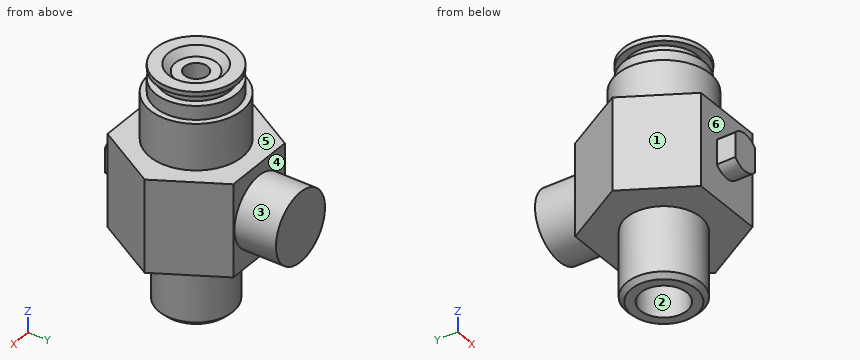
```python
from build123d import *

# Parameters (mm, degrees)
BOSS_EXTRUDE1_DEPTH = 20
SKETCH2_R           = 10
BOSS_EXTRUDE2_DEPTH = 10
SKETCH3_R           = 8.75
BOSS_EXTRUDE3_DEPTH = 6
SKETCH5_R           = 2.5
CUT_EXTRUDE1_DEPTH  = 18.5
SKETCH6_W           = 1.5
SKETCH6_H           = 2
SKETCH7_R           = 4
BOSS_EXTRUDE4_DEPTH = 4
CUT_EXTRUDE2_DEPTH  = 4
SKETCH9_R           = 7.5
BOSS_EXTRUDE5_DEPTH = 9
SKETCH10_R          = 8
SKETCH10_R_2        = 5
BOSS_EXTRUDE6_DEPTH = 15
CHAMFER1_SIZE       = 1


with BuildPart() as part:
    # Sketch1 → Boss-Extrude1 (new body)
    with BuildSketch(Plane.XY):
        Polygon((-7.875, 13.63990011), (7.875, 13.63990011), (15.75, 0), (7.875, -13.63990011), (-7.875, -13.63990011), (-15.75, 0), align=None)
    extrude(amount=BOSS_EXTRUDE1_DEPTH)

    # Sketch2 → Boss-Extrude2 (add)
    with BuildSketch(Plane.XY.offset(20)):
        Circle(SKETCH2_R)
    extrude(amount=BOSS_EXTRUDE2_DEPTH)

    # Sketch3 → Boss-Extrude3 (add)
    with BuildSketch(Plane.XY.offset(30)):
        Circle(SKETCH3_R)
    extrude(amount=BOSS_EXTRUDE3_DEPTH)

    # Sketch4 → Cut-Revolve1 (revolve, cut)
    with BuildSketch(Plane(origin=(0, 0, 0), x_dir=(1, 0, 0), z_dir=(0, 1, 0))):
        Polygon((0, -36), (-6, -36), (-4.5, -34.5), (0, -34.5), align=None)
    revolve(axis=Axis((0, 0, 45.254539395), (0, 0, -1)), mode=Mode.SUBTRACT)

    # Sketch5 → Cut-Extrude1 (cut)
    with BuildSketch(Plane.XY.offset(34.5)):
        Circle(SKETCH5_R)
    extrude(amount=-CUT_EXTRUDE1_DEPTH, mode=Mode.SUBTRACT)

    # Sketch6 → Cut-Revolve2 (revolve, cut)
    with BuildSketch(Plane(origin=(0, 0, 0), x_dir=(1, 0, 0), z_dir=(0, 1, 0))):
        with Locations((-8, -34)):
            Rectangle(SKETCH6_W, SKETCH6_H)
    revolve(axis=Axis((0, 0, 40.657268224), (0, 0, -1)), mode=Mode.SUBTRACT)

    # Sketch7 → Boss-Extrude4 (add)
    with BuildSketch(Plane.XZ.offset(13.63990011)):
        with Locations((0, 10)):
            Circle(SKETCH7_R)
    extrude(amount=BOSS_EXTRUDE4_DEPTH)

    # Sketch8 → Cut-Extrude2 (cut)
    with BuildSketch(Plane.XZ.offset(17.63990011)):
        with BuildLine():
            ThreePointArc((-3, 12.645751311), (-4, 10), (-3, 7.354248689))
            Line((-3, 7.354248689), (-3, 12.645751311))
        make_face()
        with BuildLine():
            Line((3, 12.645751311), (3, 7.354248689))
            ThreePointArc((3, 7.354248689), (3.741657387, 8.585786438), (4, 10))
            ThreePointArc((4, 10), (3.741657387, 11.414213562), (3, 12.645751311))
        make_face()
    extrude(amount=-CUT_EXTRUDE2_DEPTH, mode=Mode.SUBTRACT)

    # Sketch9 → Boss-Extrude5 (add)
    with BuildSketch(Plane(origin=(0, 13.63990011, 0), x_dir=(1, 0, 0), z_dir=(0, 1, 0))):
        with Locations((0, -10)):
            Circle(SKETCH9_R)
    extrude(amount=BOSS_EXTRUDE5_DEPTH)

    # Sketch10 → Boss-Extrude6 (add)
    with BuildSketch(Plane(origin=(0, 0, 0), x_dir=(-1, 0, 0), z_dir=(0, 0, -1))):
        Circle(SKETCH10_R)
        Circle(SKETCH10_R_2, mode=Mode.SUBTRACT)
    extrude(amount=BOSS_EXTRUDE6_DEPTH)

    # Chamfer1
    chamfer1_edges = [part.edges().sort_by_distance(p)[0] for p in [
        (8, 0, -15),
    ]]
    chamfer(chamfer1_edges, length=CHAMFER1_SIZE)


solid = part.part
```
For this review, take the finished solid that the model builds, in its own axes (mm). Face numbers are marked on the shaded views. A direction names the side the tool comes from. Round coordinates to 2 decimals unless told otherwise and drop trailing zeros. Write each loop counter-clockwise with the first axis right and the second up, starting at its lowest first coordinate (ties: lowest second). Pieces come first, ordered by that corner, then holes. Notation, with made-up numbers: (30, -30.75) - (40, -30.75) arc R27 ccw to (40, -1.75) - close; hole circle Ø7 at (83.25, 3.25). An arc over 180 degrees is marked (long way). Answer as a JSON object with one key per item and string values.
1. Draft analysis for pull direction X (two halves, no side actions). For the marked faces 1, 2 and 3, state which applies: +X half, -X half, draft (parallel to the pull), parting line (faces both ways), or undercut.
Response values:
{"face 1": "-X half", "face 2": "undercut", "face 3": "parting line"}
2. To check wall thickness, follow line 1 along Z through (x, y) = (2.5, 8); line 2 along Y through (x, z) = (0, -3.75); line 3 along Z through (x, y) = (4, 12). State the ranges of each line that lie inside material, in increasing order.
Response values:
{"line 1": "z = 0 to 33, 35 to 36", "line 2": "y = -8 to -5, 5 to 8", "line 3": "z = 0 to 20"}
3. For pin 1 Ø6 at (y, z) = (-10.5, 0) entering from +X; pin 2 Ø6 at (x, y) = (9, -7.5) entering from -Z; pin 3 Ø1.5 at (x, z) = (10, 1) entering from +Y, all flat-tipped, find the tip position at first contact; note any pin that passes through.
Response values:
{"pin 1": "stops at x = 11.42", "pin 2": "stops at z = 0", "pin 3": "stops at y = 11.26"}
4. We need section C-C on z = 26.5. Give the boundary of the cut face in (x, y).
Response values:
{"outline": "circle Ø20 at (0, 0); hole circle Ø5 at (0, 0)"}
5. We need section B-B on z = -12. Give the boundary of the cut face in (x, y), then the cut area to 3 significant figures.
Response values:
{"outline": "circle Ø16 at (0, 0); hole circle Ø10 at (0, 0)", "area": "123 mm2"}
6. Tool access review of the marked faces 4, 5 and 6: name each direction out of +Z, -Z, +X, -X, +Y, -Y from which nothing blocks a thin tool from reaching the whole face with its end or side.
Response values:
{"face 4": "+Y", "face 5": "+Z", "face 6": "-Y"}
7. We need section A-A on z = 10. Give the boundary of the cut face in (x, y) (3 decimals).
Response values:
{"outline": "(-15.75, 0) - (-7.875, -13.64) - (-3, -13.64) - (-3, -17.64) - (3, -17.64) - (3, -13.64) - (7.875, -13.64) - (15.75, 0) - (7.875, 13.64) - (7.5, 13.64) - (7.5, 22.64) - (-7.5, 22.64) - (-7.5, 13.64) - (-7.875, 13.64) - close"}
